Source: three-view drawing plus pictorial views. Frame: mm from the lowest corner of the part. A direction names the side the tool comes from. Give positions to 0.01 mm unless a question says otherwise; leave off trailing zeros. Loops run counter-clockwise (first coordinate to the right, second up) from the corner with the lowest first, then second, coordinate; pieces in that order, holes last. Notation, with made-up numbers: M -23.75,-22.5 L 35.25,-22.5 A11 ccw 35.25,-2.5 Z; hole C 86.25,-13.75 d4. An arc over 180 degrees is marked long. Put each result on its own line as item: value. Start each with the question number.
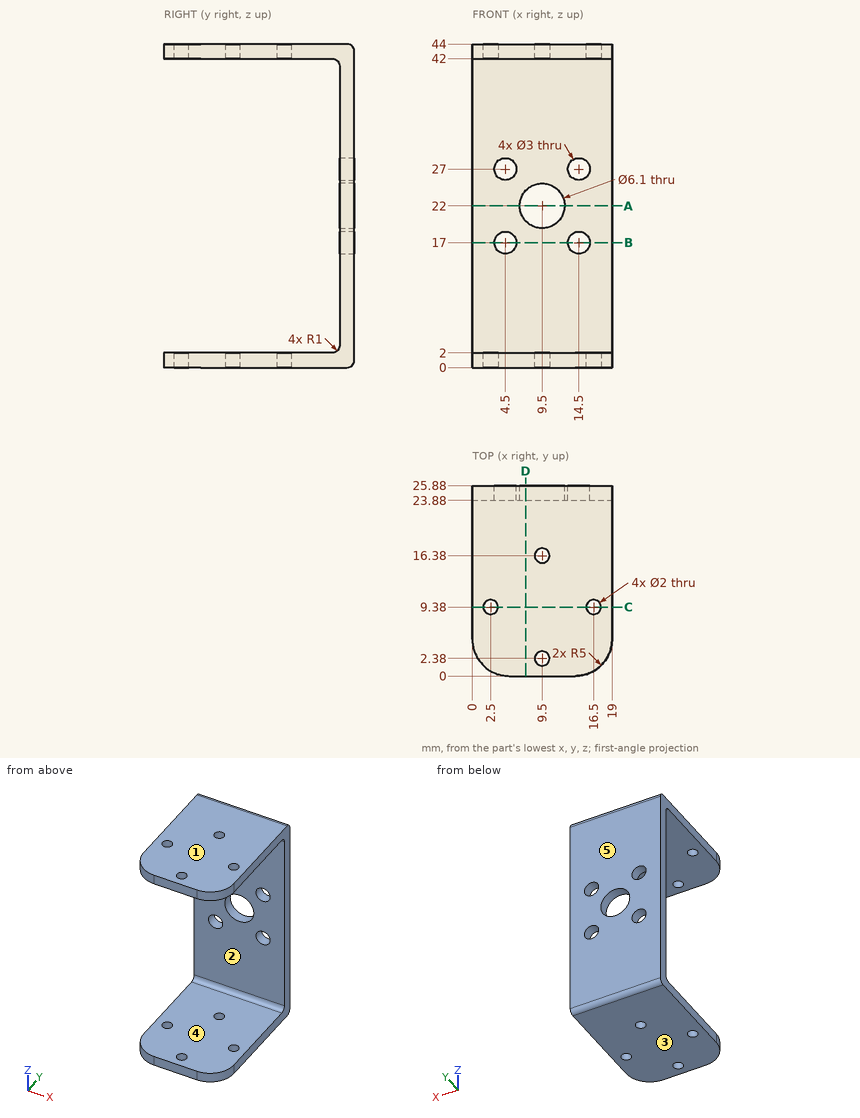
1. Section D-D, the plane x = 7.25. Output: boundary loops of the cut face in (y, z), plus the area to 3 significant figures.
2. Section B-B, the plane z = 17. Output: boundary loops of the cut face in (x, y).
3. Pull-direction query (Z, two-part tool) for the marked faces 3, 4 and 5; classes: released by +Z, released by -Z, zero draft, split by the parting line, or undercut.
4. Set-up query: the marked faces 1 and 2. Return all of +Z, -Z, +X, -X, +Y, -Y with unobstructed straight access to the full face (end or side cutting, diameter ignored); none if empty.
5. Ray query, line 1 (X direction, y = 24.65, z = 27); line 2 (Z direction, x = 6.75, y = 3.5); line 3 (Y direction, x = 12, z = 19.5). Return the intervals inside material, ascending.
6. Section C-C, the plane y = 9.38. Output: boundary loops of the cut face in (x, z), plus the area to 3 significant figures.
7. Section A-A, the plane z = 22. Output: boundary loops of the cut face in (x, y), plus the area to 3 significant figures.
8. Contact query for flat-ended pins moving along their axis: pin 1 (9.5 mm diameter, centred on x = 7, z = 21, fed in from -Y); pin 2 (2.5 mm diameter, centred on x = 4.5, z = 17, fed in from -Y). Output: stop coordinate, or through.
Results found:
1. outline: M 0,0 L 24.88,0 A1 ccw 25.88,1 L 25.88,19.94 L 23.88,19.94 L 23.88,3 A1 cw 22.88,2 L 0,2 Z; M 0,42 L 22.88,42 A1 cw 23.88,41 L 23.88,24.06 L 25.88,24.06 L 25.88,43 A1 ccw 24.88,44 L 0,44 Z
1. area: 175 mm²
2. outline: M 0,23.88 L 3,23.88 L 3,25.88 L 0,25.88 Z; M 6,23.88 L 13,23.88 L 13,25.88 L 6,25.88 Z; M 16,23.88 L 19,23.88 L 19,25.88 L 16,25.88 Z
3. face 3: released by -Z
3. face 4: undercut
3. face 5: zero draft
4. face 1: +Z, +X, -X, +Y, -Y
4. face 2: +X, -X, -Y
5. line 1: 0 to 3, 6 to 13, 16 to 19
5. line 2: 0 to 2, 42 to 44
5. line 3: 23.88 to 25.88
6. outline: M 0,0 L 1.5,0 L 1.5,2 L 0,2 Z; M 0,42 L 1.5,42 L 1.5,44 L 0,44 Z; M 3.5,0 L 15.5,0 L 15.5,2 L 3.5,2 Z; M 3.5,42 L 15.5,42 L 15.5,44 L 3.5,44 Z; M 17.5,0 L 19,0 L 19,2 L 17.5,2 Z; M 17.5,42 L 19,42 L 19,44 L 17.5,44 Z
6. area: 60.0 mm²
7. outline: M 0,23.88 L 6.45,23.88 L 6.45,25.88 L 0,25.88 Z; M 12.55,23.88 L 19,23.88 L 19,25.88 L 12.55,25.88 Z
7. area: 25.8 mm²
8. pin 1: y = 23.88
8. pin 2: through
